Can you work these out from the model? Positions are in its coordinate system, mm. A direction names the side the tool comes from. Round coordinates to 2 decimals unless told otherwise and drop trailing zeros. Write each loop counter-clockwise with the first axis right and the second up, starting at its lowest first coordinate (ties: lowest second). Pieces come first, ordered by that corner, then holes.
Q1. Please list where these lines run through material, in increasing order: line 1 along Z through (x, y) = (-5, -3.7); line 2 along X through (y, z) = (-3.5, 7).
Q2. I'm going to push a flat-ended pin straight in: pin 1 Ø12 at (x, z) = (22.5, -58.5) entering from +Y. Where does the tip first touch, or does it pass through?
Q3. If we section it at A-A (x = -48.5): Please give me the cut outline in (y, z).
Q4. For faces 4 (the flat face through (67, -2, -1)), 5 (the flat face through (77.621, -2, 2)), which set-ups out of +Z, -Z, +X, -X, +Y, -Y let a thin tool reach every point of the face, with its end or its side?
Q5. We'd pull the mould along X, two halves only. Please class faces 1 (the flat face through (-78.379, -2, 2)), 2 (the flat face through (-1, -2, -67)), 3 (the flat face through (-1, 0, 72)): +X half, -X half, draft (parallel to the pull), parting line (faces both ways), or undercut.
Q6. If we section it at B-B (z = 28.5): Please give me the cut outline in (x, y).
Q7. If we section it at C-C (y = -1.4): Please give me the cut outline in (x, z).
from build123d import *

# Parameters (mm, degrees)
F0_W     = 156
F0_H     = 156
F1_DEPTH = 4
F2_W     = 134
F2_H     = 134
F3_DEPTH = 4


with BuildPart() as f1:
    # F0 (on Front) → F1 (new body)
    with BuildSketch(Plane.XZ):
        with Locations((-0.379207, 2.60339)):
            Rectangle(F0_W, F0_H)
    extrude(amount=F1_DEPTH)

    # F2 (on face) → F3 (cut)
    with BuildSketch(Plane.XZ.offset(4)):
        Rectangle(F2_W, F2_H)
    extrude(amount=-F3_DEPTH, mode=Mode.SUBTRACT)


solid = f1.part
A:
1. line 1: z = -75.4 to -67, 67 to 80.6
1. line 2: x = -78.38 to -67, 67 to 77.62
2. pin 1: passes through
3. outline: (-4, -75.4) - (0, -75.4) - (0, -67) - (-4, -67) - close; (-4, 67) - (0, 67) - (0, 80.6) - (-4, 80.6) - close
4. face 4: +Y, -Y
4. face 5: +Z, -Z, +X, +Y, -Y
5. face 1: -X half
5. face 2: undercut
5. face 3: draft
6. outline: (-78.38, -4) - (-67, -4) - (-67, 0) - (-78.38, 0) - close; (67, -4) - (77.62, -4) - (77.62, 0) - (67, 0) - close
7. outline: (-78.38, -75.4) - (77.62, -75.4) - (77.62, 80.6) - (-78.38, 80.6) - close; hole (-67, -67) - (67, -67) - (67, 67) - (-67, 67) - close
